Design review of the part built by this model. Coordinates are the model's own, in mm. A direction names the side the tool comes from. Coordinates: 2 decimals unless noted, no trailing zeros. Loops run counter-clockwise (first coordinate to the right, second up) from the corner with the lowest first, then second, coordinate; pieces in that order, holes last. Notation, with made-up numbers: (6, 38.5) -> (42, 38.5) arc R29 cw to (42, 62.5) -> close; hole circle Ø5 at (9.5, 35.5). An arc over 180 degrees is marked (long way). Use a Markdown table: item, result. Add a question column.
Q1. For probe 1 along X at (y, z) = (2.5, 1); probe 2 along Z at (x, y) = (-2, 0.25); probe 3 along Y at (x, z) = (1, 12.5), list the stretches that pass through material, from the lowest coordinate up.
Q2. Take a section at D-D on z = 9.25. Write out the cut boundary in (x, y), plus the area to 3 significant figures.
Q3. Take a section at C-C on x = 8. Write out the cut boundary in (y, z), plus the area to 3 significant figures.
Q4. Draft analysis for pull direction X (two halves, no side actions). For faces 1 (the face through (-9, -3, 2)), 2 (the face through (8, 2, -8)), 3 (the face through (9, -3, 0)), 4 (the face through (4.5, 3, 11)), state which applies: pulls with the +X half, pulls with the -X half, needs draft (parallel to the pull), parting line crosses it, or undercut.
Q5. Take a section at B-B on z = 3.75. Write out the cut boundary in (x, y).
Q6. For faces 5 (the face through (-8, 2, -8)), 6 (the face through (0, 1, 13)), 7 (the face through (8, 3, 2)), 8 (the face through (6.5, 2, 2)), 9 (the face through (8, -4, -8)), list the 3-axis set-ups (+Z, -Z, +X, -X, +Y, -Y) from which the entire face can be reached by the end or side of a thin tool; tool diameter is ignored.
Q7. Clearance check with flat-ended pins moving along their axes: pin 1 Ø6 at (x, y) = (1, -1) entering from +Z; pin 2 Ø1.2 at (x, z) = (-8.5, 6.5) entering from +Y; pin 3 Ø0.8 at (x, y) = (-7.5, -3.5) entering from -Z; pin 4 Ø2.5 at (x, z) = (-1.5, 14) entering from -Y. State where each tip first meets the part, or that it passes through.
Q8. Take a section at A-A on y = -3.75. Write out the cut boundary in (x, z), plus the area to 3 significant figures.
from build123d import *

# Parameters (mm, degrees)
SKETCH_1_W           = 18
SKETCH_1_H           = 24
EXTRUDE_1_DEPTH      = 1
SKETCH_2_W           = 9
SKETCH_2_H           = 7.4
EXTRUDE_2_DEPTH      = 3.3
EXTRUDE_3_DEPTH      = 9
EXTRUDE_3_DEPTH_BACK = 3
SKETCH_3_W           = 2.5
SKETCH_3_H           = 20


with BuildPart() as part:
    # 草图1 → 凸台-拉伸1 (new body)
    with BuildSketch(Plane(origin=(0, 0, 0), x_dir=(1, 0, 0), z_dir=(0, 1, 0))):
        Rectangle(SKETCH_1_W, SKETCH_1_H)
    extrude(amount=EXTRUDE_1_DEPTH)

    # 草图2 → 凸台-拉伸2 (add)
    with BuildSketch(Plane(origin=(0, 1, 0), x_dir=(1, 0, 0), z_dir=(0, 1, 0))):
        with Locations((0, -11.3)):
            Rectangle(SKETCH_2_W, SKETCH_2_H)
    extrude(amount=EXTRUDE_2_DEPTH)

    # 草图3 → 凸台-拉伸3 (add, two sides: drawn at the far end of the back side and taken through both)
    with BuildSketch(Plane.XZ.offset(-EXTRUDE_3_DEPTH_BACK)):
        with Locations((-7.75, 2)):
            Rectangle(SKETCH_3_W, SKETCH_3_H)
        with Locations((7.75, 2)):
            Rectangle(SKETCH_3_W, SKETCH_3_H)
    extrude(amount=EXTRUDE_3_DEPTH + EXTRUDE_3_DEPTH_BACK)


solid = part.part
Answer list:
| question | item | result |
|---|---|---|
| 1 | probe 1 | -9 to -6.5, 6.5 to 9 |
| 1 | probe 2 | -12 to 12 |
| 1 | probe 3 | 1 to 4.3 |
| 2 | outline | (-9, -9) -> (-6.5, -9) -> (-6.5, 0) -> (6.5, 0) -> (6.5, -9) -> (9, -9) -> (9, 3) -> (6.5, 3) -> (6.5, 1) -> (4.5, 1) -> (4.5, 4.3) -> (-4.5, 4.3) -> (-4.5, 1) -> (-6.5, 1) -> (-6.5, 3) -> (-9, 3) -> close |
| 2 | area | 103 mm² |
| 3 | outline | (-9, -8) -> (0, -8) -> (0, -12) -> (1, -12) -> (1, -8) -> (3, -8) -> (3, 12) -> (-9, 12) -> close |
| 3 | area | 244 mm² |
| 4 | face 1 | pulls with the -X half |
| 4 | face 2 | needs draft |
| 4 | face 3 | pulls with the +X half |
| 4 | face 4 | undercut |
| 5 | outline | (-9, -9) -> (-6.5, -9) -> (-6.5, 0) -> (6.5, 0) -> (6.5, -9) -> (9, -9) -> (9, 3) -> (6.5, 3) -> (6.5, 1) -> (-6.5, 1) -> (-6.5, 3) -> (-9, 3) -> close |
| 6 | face 5 | -Z, +X, -X, +Y |
| 6 | face 6 | +Z, +X, -X, -Y |
| 6 | face 7 | +Z, -Z, +X, +Y |
| 6 | face 8 | +Z, -Z, +Y |
| 6 | face 9 | -Z, +X, -X, -Y |
| 7 | pin 1 | z = 15 |
| 7 | pin 2 | y = 3 |
| 7 | pin 3 | z = -8 |
| 7 | pin 4 | y = 1 |
| 8 | outline | (-9, -8) -> (-6.5, -8) -> (-6.5, 12) -> (-9, 12) -> close; (6.5, -8) -> (9, -8) -> (9, 12) -> (6.5, 12) -> close |
| 8 | area | 100 mm² |
